Print and shaded views of the part. All mm, measured from the part's lowest x, y and z. A direction names the side the tool comes from. Give positions to 0.01 mm unless a question says otherwise; leave off trailing zeros. Loops run counter-clockwise (first coordinate to the right, second up) from the corner with the lowest first, then second, coordinate; pieces in that order, holes last. Notation, with made-up numbers: M 79.25,58.5 L 102.25,58.5 A11 ccw 102.25,62.5 Z; hole C 23.25,30.25 d4. An arc over 180 degrees is marked long. Answer as CSV lines item,"result".
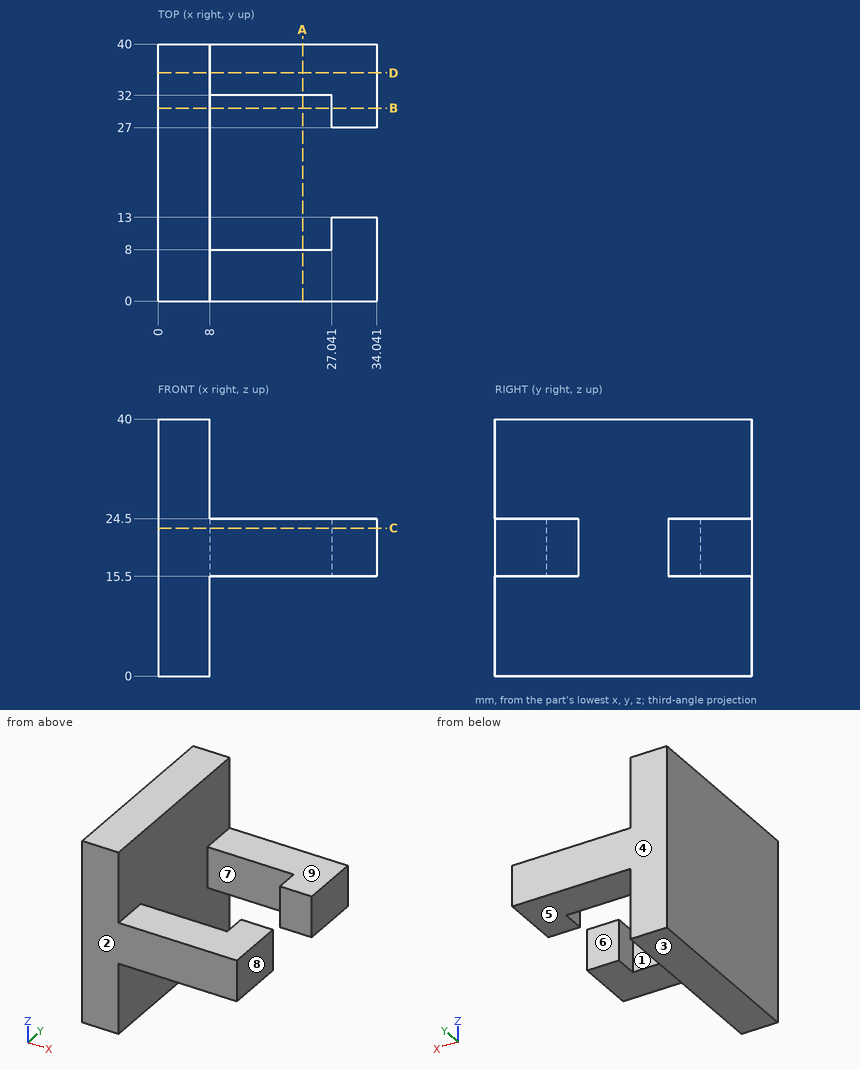
Q1. Mould opens along Y. For the marked faces 1, 2, 3 and 4 say: released by +Y, released by -Y, zero draft, split by the parting line, or undercut.
Solution:
face 1,"undercut"
face 2,"released by -Y"
face 3,"zero draft"
face 4,"released by +Y"
Q2. Cut at C-C (z = 23). Write the cut outline in (x, y).
Solution:
outline,"M 0,0 L 34.04,0 L 34.04,13 L 27.04,13 L 27.04,8 L 8,8 L 8,32 L 27.04,32 L 27.04,27 L 34.04,27 L 34.04,40 L 0,40 Z"
Q3. Pin check, flat tips, straight feed: P1, Ø10.5, axis at x = 17, y = 32.5, coming from the +Z side; P2, Ø12, axis at y = 20.5, z = 24, coming from the +X side; P3, Ø14.5, axis at x = 16.5, y = 35, coming from the -Z side. Stop position of each tip, or through.
Solution:
P1,"stops at z = 24.5"
P2,"stops at x = 8"
P3,"stops at z = 15.5"
Q4. Wall check: line 1 (Y direction, x = 11.5, z = 19.5); line 2 (X direction, y = 28, z = 6.5); line 3 (Z direction, x = 22, y = 34). Give the ranges that are in metal, low to high. Write a range as [from, to].
Solution:
line 1,"y = [0, 8], [32, 40]"
line 2,"x = [0, 8]"
line 3,"z = [15.5, 24.5]"
Q5. Cut at B-B (y = 30). Write the cut outline in (x, z), and give its area (3 significant figures).
Solution:
outline,"M 0,0 L 8,0 L 8,40 L 0,40 Z; M 27.04,15.5 L 34.04,15.5 L 34.04,24.5 L 27.04,24.5 Z"
area,"383 mm²"
Q6. Cut at D-D (y = 35.5). Write the cut outline in (x, z).
Solution:
outline,"M 0,0 L 8,0 L 8,15.5 L 34.04,15.5 L 34.04,24.5 L 8,24.5 L 8,40 L 0,40 Z"
Q7. Which spindle directions (+Z, -Z, +X, -X, +Y, -Y) get a long thin tool onto all of the face, cutting with end or side? Do the marked faces 5, 6, 7, 8 and 9. Say none if no direction does.
Solution:
face 5,"-Z, +X, +Y, -Y"
face 6,"+Z, -Z, +X"
face 7,"+Z, -Z"
face 8,"+Z, -Z, +X, +Y, -Y"
face 9,"+Z, +X, +Y, -Y"
Q8. Cut at A-A (x = 22.5). Write the cut outline in (y, z), and give its area (3 significant figures).
Solution:
outline,"M 0,15.5 L 8,15.5 L 8,24.5 L 0,24.5 Z; M 32,15.5 L 40,15.5 L 40,24.5 L 32,24.5 Z"
area,"144 mm²"
